from build123d import *

# Parameters (mm, degrees)
F0_W     = 144
F0_H     = 72
F1_DEPTH = 2


with BuildPart() as f1:
    # F0 (on Right) → F1 (new body)
    with BuildSketch(Plane.YZ):
        with Locations((72, 36)):
            Rectangle(F0_W, F0_H)
        Polygon((139.711167, 2), (2, 2), (2, 68.888281), align=None, mode=Mode.SUBTRACT)
        Polygon((4.288833, 70), (142, 70), (142, 3.111719), align=None, mode=Mode.SUBTRACT)
    extrude(amount=F1_DEPTH)


solid = f1.part
Part model, mm, in its own coordinate system. A direction names the side the tool comes from. Round coordinates to 2 decimals unless told otherwise and drop trailing zeros. Write each loop counter-clockwise with the first axis right and the second up, starting at its lowest first coordinate (ties: lowest second). Pieces come first, ordered by that corner, then holes. Notation, with made-up numbers: M 8.5,49 L 43.5,49 A17 ccw 43.5,60 Z; hole C 82.25,4 d8. An arc over 180 degrees is marked long. Return JSON: item names as keys, results as strings. Group by question number.
(1) Which spindle directions (+Z, -Z, +X, -X, +Y, -Y) get a long thin tool onto all of the face, cutting with end or side? Do faces 1 (the face through (2, 72, 36)), 2 (the face through (0.986, 74.108, 36.088)). Say none if no direction does.
(2) Saw through at C-C on z = 50. Write the cut outline in (x, y), then the cut area to 3 significant figures.
(3) Two-plate mould, pull along Z, no slides. Class faces 3 (the face through (0.986, 69.892, 35.912)), 4 (the face through (0, 72, 36)): +Z half, -Z half, draft (parallel to the pull), parting line (faces both ways), or undercut.
(4) Saw through at A-A on x = 0.6. Write the cut outline in (y, z).
(5) Drill centre lines: probe 1 along Y at (x, z) = (1, 9.5); probe 2 along Z at (x, y) = (1.9, 31.5); probe 3 along Y at (x, z) = (1.4, 35). Where is each one in solid material? Low to high.
(6) Saw through at B-B on y = 67. Write the cut outline in (x, z).
Returned:
{
 "1": {"face 1": "+Z, -Z, +X, +Y, -Y", "face 2": "+X, -X"},
 "2": {"outline": "M 0,0 L 2,0 L 2,2 L 0,2 Z; M 0,40.89 L 2,40.89 L 2,45.47 L 0,45.47 Z; M 0,142 L 2,142 L 2,144 L 0,144 Z", "area": "17.2 mm²"},
 "3": {"face 3": "undercut", "face 4": "draft"},
 "4": {"outline": "M 0,0 L 144,0 L 144,72 L 0,72 Z; hole M 2,2 L 139.71,2 L 2,68.89 Z; hole M 4.29,70 L 142,3.11 L 142,70 Z"},
 "5": {"probe 1": "0 to 2, 124.27 to 128.85, 142 to 144", "probe 2": "0 to 2, 54.56 to 56.78, 70 to 72", "probe 3": "0 to 2, 71.77 to 76.35, 142 to 144"},
 "6": {"outline": "M 0,0 L 2,0 L 2,2 L 0,2 Z; M 0,37.32 L 2,37.32 L 2,39.54 L 0,39.54 Z; M 0,70 L 2,70 L 2,72 L 0,72 Z"}
}
